```python
from build123d import *

# Parameters (mm, degrees)
SKETCH1_R           = 1.524
SKETCH1_R_2         = 1.5875
SKETCH1_R_3         = 5.461
BOSS_EXTRUDE1_DEPTH = 3.175


with BuildPart() as part:
    # Sketch1 → Boss-Extrude1 (new body)
    with BuildSketch(Plane.XY):
        Polygon((-24.889290425, 17.419992315), (0.510709575, 17.419992315), (0.510709575, 14.244992315), (25.910709575, 14.244992315), (25.910709575, 17.419992315), (51.310709575, 17.419992315), (51.310709575, 14.244992315), (76.710709575, 14.244992315), (76.710709575, 17.419992315), (102.110709575, 17.419992315), (102.110709575, 14.244992315), (152.910709575, 14.244992315), (162.435709575, 14.244992315), (162.435709575, -23.855007685), (102.110709575, -23.855007685), (102.110709575, -27.030007685), (76.710709575, -27.030007685), (76.710709575, -23.855007685), (51.310709575, -23.855007685), (51.310709575, -27.030007685), (25.910709575, -27.030007685), (25.910709575, -23.855007685), (0.510709575, -23.855007685), (0.510709575, -27.030007685), (-24.889290425, -27.030007685), (-24.889290425, -23.855007685), (-50.289290425, -23.855007685), (-50.289290425, -27.030007685), (-75.689290425, -27.030007685), (-75.689290425, 17.419992315), (-50.289290425, 17.419992315), (-50.289290425, 14.244992315), (-24.889290425, 14.244992315), align=None)
        with Locations((-47.139690425, -4.805007685)):
            Circle(SKETCH1_R, mode=Mode.SUBTRACT)
        with Locations((-56.639290425, -12.806007685)):
            Circle(SKETCH1_R, mode=Mode.SUBTRACT)
        with Locations((-56.639290425, 3.195992315)):
            Circle(SKETCH1_R, mode=Mode.SUBTRACT)
        with Locations((-66.138890425, -4.805007685)):
            Circle(SKETCH1_R, mode=Mode.SUBTRACT)
        with Locations((157.673209575, -4.805007685)):
            Circle(SKETCH1_R_2, mode=Mode.SUBTRACT)
        with Locations((-56.639290425, -4.805007685)):
            Circle(SKETCH1_R_3, mode=Mode.SUBTRACT)
        with BuildLine():
            Line((-2.448912015, -0.76389243), (1.873921506, 3.558941091))
            ThreePointArc((1.873921506, 3.558941091), (2.424524294, 6.327008233), (0.077870282, 7.894992315))
            Line((0.077870282, 7.894992315), (-8.567796761, 7.894992315))
            ThreePointArc((-8.567796761, 7.894992315), (-10.914450773, 6.327008233), (-10.363847985, 3.558941091))
            Line((-10.363847985, 3.558941091), (-6.041014464, -0.76389243))
            ThreePointArc((-6.041014464, -0.76389243), (-4.244963239, -1.507841206), (-2.448912015, -0.76389243))
        make_face(mode=Mode.SUBTRACT)
        with BuildLine():
            Line((-8.567796761, -17.505007685), (0.077870282, -17.505007685))
            ThreePointArc((0.077870282, -17.505007685), (2.424524294, -15.937023603), (1.873921506, -13.168956461))
            Line((1.873921506, -13.168956461), (-2.448912015, -8.846122939))
            ThreePointArc((-2.448912015, -8.846122939), (-4.244963239, -8.102174164), (-6.041014464, -8.846122939))
            Line((-6.041014464, -8.846122939), (-10.363847985, -13.168956461))
            ThreePointArc((-10.363847985, -13.168956461), (-10.914450773, -15.937023603), (-8.567796761, -17.505007685))
        make_face(mode=Mode.SUBTRACT)
        with BuildLine():
            Line((-37.589290425, 5.354992315), (-37.589290425, -14.965007685))
            ThreePointArc((-37.589290425, -14.965007685), (-36.845341649, -16.761058909), (-35.049290425, -17.505007685))
            Line((-35.049290425, -17.505007685), (-20.242129718, -17.505007685))
            ThreePointArc((-20.242129718, -17.505007685), (-19.2701138, -17.311661697), (-18.446078494, -16.761058909))
            Line((-18.446078494, -16.761058909), (-8.286078494, -6.601058909))
            ThreePointArc((-8.286078494, -6.601058909), (-7.542129718, -4.805007685), (-8.286078494, -3.008956461))
            Line((-8.286078494, -3.008956461), (-18.446078494, 7.151043539))
            ThreePointArc((-18.446078494, 7.151043539), (-19.2701138, 7.701646328), (-20.242129718, 7.894992315))
            Line((-20.242129718, 7.894992315), (-35.049290425, 7.894992315))
            ThreePointArc((-35.049290425, 7.894992315), (-36.845341649, 7.151043539), (-37.589290425, 5.354992315))
        make_face(mode=Mode.SUBTRACT)
        with BuildLine():
            Line((9.956152015, 7.151043539), (-0.203847985, -3.008956461))
            ThreePointArc((-0.203847985, -3.008956461), (-0.947796761, -4.805007685), (-0.203847985, -6.601058909))
            Line((-0.203847985, -6.601058909), (9.956152015, -16.761058909))
            ThreePointArc((9.956152015, -16.761058909), (10.780187321, -17.311661697), (11.752203239, -17.505007685))
            Line((11.752203239, -17.505007685), (20.677590576, -17.505007685))
            ThreePointArc((20.677590576, -17.505007685), (21.649606495, -17.311661697), (22.473641801, -16.761058909))
            Line((22.473641801, -16.761058909), (42.793641801, 3.558941091))
            ThreePointArc((42.793641801, 3.558941091), (43.344244589, 6.327008233), (40.997590576, 7.894992315))
            Line((40.997590576, 7.894992315), (11.752203239, 7.894992315))
            ThreePointArc((11.752203239, 7.894992315), (10.780187321, 7.701646328), (9.956152015, 7.151043539))
        make_face(mode=Mode.SUBTRACT)
        with BuildLine():
            Line((121.067497644, -16.761058909), (110.907497644, -6.601058909))
            ThreePointArc((110.907497644, -6.601058909), (110.163548868, -4.805007685), (110.907497644, -3.008956461))
            Line((110.907497644, -3.008956461), (121.067497644, 7.151043539))
            ThreePointArc((121.067497644, 7.151043539), (121.89153295, 7.701646328), (122.863548868, 7.894992315))
            Line((122.863548868, 7.894992315), (137.670709575, 7.894992315))
            ThreePointArc((137.670709575, 7.894992315), (139.466760799, 7.151043539), (140.210709575, 5.354992315))
            Line((140.210709575, 5.354992315), (140.210709575, -14.965007685))
            ThreePointArc((140.210709575, -14.965007685), (139.466760799, -16.761058909), (137.670709575, -17.505007685))
            Line((137.670709575, -17.505007685), (122.863548868, -17.505007685))
            ThreePointArc((122.863548868, -17.505007685), (121.89153295, -17.311661697), (121.067497644, -16.761058909))
        make_face(mode=Mode.SUBTRACT)
        with BuildLine():
            Line((90.869215911, 7.894992315), (61.623828574, 7.894992315))
            ThreePointArc((61.623828574, 7.894992315), (59.277174561, 6.327008233), (59.82777735, 3.558941091))
            Line((59.82777735, 3.558941091), (80.14777735, -16.761058909))
            ThreePointArc((80.14777735, -16.761058909), (80.971812656, -17.311661697), (81.943828574, -17.505007685))
            Line((81.943828574, -17.505007685), (90.869215911, -17.505007685))
            ThreePointArc((90.869215911, -17.505007685), (91.841231829, -17.311661697), (92.665267135, -16.761058909))
            Line((92.665267135, -16.761058909), (102.825267135, -6.601058909))
            ThreePointArc((102.825267135, -6.601058909), (103.569215911, -4.805007685), (102.825267135, -3.008956461))
            Line((102.825267135, -3.008956461), (92.665267135, 7.151043539))
            ThreePointArc((92.665267135, 7.151043539), (91.841231829, 7.701646328), (90.869215911, 7.894992315))
        make_face(mode=Mode.SUBTRACT)
        with BuildLine():
            Line((111.189215911, -17.505007685), (102.543548868, -17.505007685))
            ThreePointArc((102.543548868, -17.505007685), (100.196894856, -15.937023603), (100.747497644, -13.168956461))
            Line((100.747497644, -13.168956461), (105.070331165, -8.846122939))
            ThreePointArc((105.070331165, -8.846122939), (106.86638239, -8.102174164), (108.662433614, -8.846122939))
            Line((108.662433614, -8.846122939), (112.985267135, -13.168956461))
            ThreePointArc((112.985267135, -13.168956461), (113.535869924, -15.937023603), (111.189215911, -17.505007685))
        make_face(mode=Mode.SUBTRACT)
        with BuildLine():
            Line((105.070331165, -0.76389243), (100.747497644, 3.558941091))
            ThreePointArc((100.747497644, 3.558941091), (100.196894856, 6.327008233), (102.543548868, 7.894992315))
            Line((102.543548868, 7.894992315), (111.189215911, 7.894992315))
            ThreePointArc((111.189215911, 7.894992315), (113.535869924, 6.327008233), (112.985267135, 3.558941091))
            Line((112.985267135, 3.558941091), (108.662433614, -0.76389243))
            ThreePointArc((108.662433614, -0.76389243), (106.86638239, -1.507841206), (105.070331165, -0.76389243))
        make_face(mode=Mode.SUBTRACT)
        with BuildLine():
            Line((67.742713319, -8.846122939), (72.065546841, -13.168956461))
            ThreePointArc((72.065546841, -13.168956461), (72.616149629, -15.937023603), (70.269495616, -17.505007685))
            Line((70.269495616, -17.505007685), (32.351923534, -17.505007685))
            ThreePointArc((32.351923534, -17.505007685), (30.005269521, -15.937023603), (30.55587231, -13.168956461))
            Line((30.55587231, -13.168956461), (49.514658351, 5.789829581))
            ThreePointArc((49.514658351, 5.789829581), (51.310709575, 6.533778356), (53.106760799, 5.789829581))
            Line((53.106760799, 5.789829581), (67.742713319, -8.846122939))
        make_face(mode=Mode.SUBTRACT)
    extrude(amount=BOSS_EXTRUDE1_DEPTH)


solid = part.part
```
Verification items for the finished model (mm, model axes). A direction names the side the tool comes from. Coordinates: 2 decimals unless noted, no trailing zeros. Order: outer loops, then holes, each group sorted by start corner. A loop starts at its lowest first (then second) coordinate and runs counter-clockwise, first axis right, second up. Notation, with made-up numbers: (81, 34) -> (123, 34) arc R16 cw to (123, 46) -> close; hole circle Ø2 at (47.5, 89.25). An arc over 180 degrees is marked (long way). Answer as CSV lines item,"result". Start each with the question number.
1) Gauge pin test, flat ends, axial feed: pin 1 Ø12 at (x, y) = (126.5, -6) entering from +Z; pin 2 Ø1.6 at (x, z) = (105.5, 2) entering from -Y (3 decimals); pin 3 Ø1 at (y, z) = (-24.5, 1.5) entering from +X; pin 4 Ø1 at (x, z) = (61, 1) entering from +Y (3 decimals). Record the tip position at first contact, or that the pin passes through.
2) Release check for a two-part mould opening along Y. For faces 1 (the face through (45, 5, 3.175)), 2 (the face through (110.794, -10.977, 1.565)) record: released by +Y, released by -Y, zero draft, split by the parting line, or undercut.
3) Cross-section at B-B, the plane z = 1.15. Give the number of separate pieces and of enclosed holes in the cut face, then the cut area to 3 significant figures.
4) Material ranges on L1, parallel to X at y = 15.5, z = 1.1; L2, parallel to Y at x = -1, z = 2.05 (3 decimals); L3, parallel to Y at x = 85, z = 0.6 (3 decimals), recorded low to high. Write a range as [from, to].
5) Cross-section at A-A, the plane x = 14. Record the boundary of the cut face in (y, z) (3 decimals), then the cut area to 3 significant figures.
6) Set-up check for faces 3 (the face through (32.491, -6.743, 1.565)), 4 (the face through (45, 5, 0)): record each of +Z, -Z, +X, -X, +Y, -Y from which the full face is reachable in a straight line by a thin tool's end or side.
Conclusion:
1,pin 1,"passes through"
1,pin 2,"stops at y = -23.855"
1,pin 3,"stops at x = 102.11"
1,pin 4,"stops at y = 14.245"
2,face 1,"zero draft"
2,face 2,"undercut"
3,separate pieces,"1"
3,enclosed holes,"15"
3,area,"5,850 mm²"
4,L1,"x = [-75.69, -50.29], [-24.89, 0.51], [25.91, 51.31], [76.71, 102.11]"
4,L2,"y = [-27.03, -17.505], [-10.295, 0.685], [7.895, 17.42]"
4,L3,"y = [-27.03, -17.505], [7.895, 17.42]"
5,outline,"(-23.855, 0) -> (-17.505, 0) -> (-17.505, 3.175) -> (-23.855, 3.175) -> close; (7.895, 0) -> (14.245, 0) -> (14.245, 3.175) -> (7.895, 3.175) -> close"
5,area,"40.3 mm²"
6,face 3,"+Z, -Z"
6,face 4,"-Z, +X, -X, +Y, -Y"
